Autodesk Inventor part; units mm, degrees
ref_plane "YZ Plane" through (0, 0, 0) normal (1, 0, 0) x (0, 1, 0)
ref_plane "XZ Plane" through (0, 0, 0) normal (0, 1, 0) x (-1, 0, 0)
ref_plane "XY Plane" through (0, 0, 0) normal (0, 0, 1) x (1, 0, 0)
ref_plane "Plano de trabajo1" through (0, 0, 0) normal (0, 0, 1) x (1, 0, 0)
sketch "Boceto1" plane through (0, 0, 0) normal (0, 0, 1) x (1, 0, 0)
  circle A0 centre (70, 9.3) radius 2.5
  circle A1 centre (10, 9.3) radius 2.5
  arc A2 (80, 12) -> (77, 15) centre (77, 12) ccw
  line L0 (3, 15) -> (77, 15)
  arc A3 (3, 15) -> (0, 12) centre (3, 12) ccw
  line L1 (0, 12) -> (0, -2)
  line L2 (0, -2) -> (0.1716, -2)
  arc A4 (3, 0) -> (0.1716, -2) centre (3, -3) ccw
  line L3 (77, 0) -> (3, 0)
  arc A5 (79.8284, -2) -> (77, 0) centre (77, -3) ccw
  line L4 (79.8284, -2) -> (80, -2)
  line L5 (80, -2) -> (80, 12)
  line L6 (0, 0) -> (80, 0)
  line L7 (80, 0) -> (80, 25)
  line L8 (80, 25) -> (0, 25)
  line L9 (0, 25) -> (0, 0)
  point P0 (0, 12)
  dimension "d0" = 25
extrude "Extrusión1" add sketch "Boceto1" along normal blind 2 contours A0 | A1 | L5 L6 L3 L1 A3 L0 A2 | A2 L0 A3 L9 L8 L7
sketch "Boceto2" plane through (0, 0, 0) normal (0, 0, -1) x (-1, 0, 0)
  circle A0 centre (-10, 9.3) radius 2.5
  circle A1 centre (-70, 9.3) radius 2.5
  line L0 (-10, 9.3) -> (-10, 19.3)
  line L1 (-70, 9.3) -> (-70, 19.3)
  point P0 (0, 0)
  dimension "d3" = 10
  dimension "d4" = 10
sketch "Boceto3" plane through (0, 0, 0) normal (0, 0, -1) x (-1, 0, 0)
  arc A0 (-77, 15) -> (-80, 12) centre (-77, 12) ccw
  line L0 (-80, -2) -> (-80, 12)
  line L1 (-80, -2) -> (0, -2)
  line L2 (0, -2) -> (0, 12)
  arc A1 (0, 12) -> (-3, 15) centre (-3, 12) ccw
  line L3 (-77, 15) -> (-3, 15)
  circle A2 centre (-70, 9.3) radius 2.5
  circle A3 centre (-10, 9.3) radius 2.5
  line L4 (-80, 25) -> (0, 25)
  line L5 (-80, 0) -> (-80, 25)
  line L6 (0, 0) -> (-80, 0)
  line L7 (0, 25) -> (0, 0)
  line L8 (-80, 25) -> (0, 25)
  line L9 (0, 25) -> (0, 15)
  line L10 (0, 15) -> (-80, 15)
  line L11 (-80, 15) -> (-80, 25)
  point P0 (-77, 15)
  point P1 (-3, 15)
  dimension "d14" = 10
extrude "Extrusión2" add sketch "Boceto3" along normal blind 3 contours L10 L5 L4 L7 L3
hole "Agujero1" at (70, 19.3, 0) at (10, 19.3, 0) direction (0, 0, 1) diameter 5 end through all both
properties part number "Adaptador"
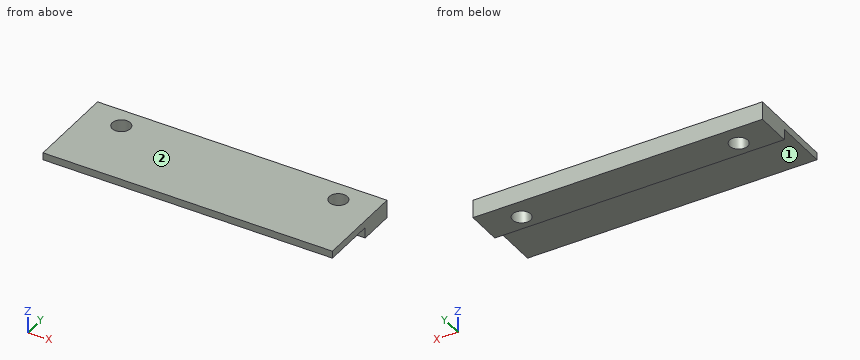
Geometry check sheet. Reference: the model listing, model coordinates, mm. Face numbers are marked on the shaded views. A direction names the side the tool comes from. Round coordinates to 2 decimals unless told otherwise and drop trailing zeros. Order: outer loops, then holes, each group sorted by start corner. A loop starts at its lowest first (then second) coordinate and runs counter-clockwise, first axis right, second up. Notation, with made-up numbers: M -27.5,41.25 L -13.5,41.25 A12 ccw -13.5,61.25 Z; hole C -18,35 d8. An arc over 180 degrees is marked long. Answer in a Markdown table with one row per item.
(1) Go/stop test with flat-tipped pins: P1, Ø10, axis at x = 65, y = 3.5, coming from the -Z side; P2, Ø0.9, axis at x = 51, z = -2, coming from the -Y side. Record where each tip stops, or that it passes through.
Responses:
| item | result |
|---|---|
| P1 | stops at z = 0 |
| P2 | stops at y = 15 |
(2) Scan lines: probe 1 along X at (y, z) = (19.3, -1.15); probe 2 along X at (y, z) = (17, 1.45); probe 3 along Y at (x, z) = (10, -2). Record each from-to range of solid material in increasing order. Write a range as from..to.
Responses:
| item | result |
|---|---|
| probe 1 | x = 0..7.5, 12.5..67.5, 72.5..80 |
| probe 2 | x = 0..9.02, 10.98..69.02, 70.98..80 |
| probe 3 | y = 15..16.8, 21.8..25 |
(3) Tool access check on the marked faces 1 and 2. Record the directions out of +Z, -Z, +X, -X, +Y, -Y that give a thin tool (end or side, any length) a straight path to the whole face; none if there is none.
Responses:
| item | result |
|---|---|
| face 1 | -Z, +X, -X, -Y |
| face 2 | +Z, +X, -X, +Y, -Y |
(4) Sectioned sample at C-C, the plane y = 20. Record the cut outline in (x, z).
Responses:
| item | result |
|---|---|
| outline | M 0,-3 L 7.6,-3 L 7.6,2 L 0,2 Z; M 12.4,-3 L 67.6,-3 L 67.6,2 L 12.4,2 Z; M 72.4,-3 L 80,-3 L 80,2 L 72.4,2 Z |
(5) Sectioned sample at D-D, the plane y = 12. Record the cut outline in (x, z).
Responses:
| item | result |
|---|---|
| outline | M 0,0 L 80,0 L 80,2 L 0,2 Z |
(6) Sectioned sample at A-A, the plane x = 70. Record the cut outline in (y, z).
Responses:
| item | result |
|---|---|
| outline | M 0,0 L 15,0 L 15,-3 L 16.8,-3 L 16.8,2 L 0,2 Z; M 21.8,-3 L 25,-3 L 25,2 L 21.8,2 Z |
(7) Sectioned sample at B-B, the plane z = 1.15. Record the cut outline in (x, y), and give its area (3 significant figures).
Responses:
| item | result |
|---|---|
| outline | M 0,0 L 80,0 L 80,25 L 0,25 Z; hole C 10,19.3 d5; hole C 70,19.3 d5 |
| area | 1,960 mm² |
